Build history of the part. All positions in model axes, mm. A direction names the side the tool comes from. Give positions to 0.01 mm unless a question says otherwise; leave off trailing zeros. Order: outer loops, then holes, each group sorted by start corner. A loop starts at its lowest first (then second) coordinate and runs counter-clockwise, first axis right, second up. Notation, with made-up numbers: M -33,-30.5 L -15,-30.5 A28 ccw -15,-0.5 Z; hole C -22,57 d2. An arc over 180 degrees is marked long. One line per item, written item: value.
from build123d import *

# Parameters (mm, degrees)
BOSS_EXTRUDE1_DEPTH = 340


with BuildPart() as part:
    # Sketch1 → Boss-Extrude1 (new body)
    with BuildSketch(Plane(origin=(0, 0, 0), x_dir=(1, 0, 0), z_dir=(0, 1, 0))):
        with BuildLine():
            Line((-27.499872145, 29.213153277), (-67.499872145, 29.213153277))
            Line((-67.499872145, 29.213153277), (-67.499872145, -10.786846723))
            Line((-67.499872145, -10.786846723), (-66.499872145, -10.786846723))
            ThreePointArc((-66.499872145, -10.786846723), (-64.378551801, -9.908167067), (-63.499872145, -7.786846723))
            Line((-63.499872145, -7.786846723), (-63.499872145, 22.213153277))
            ThreePointArc((-63.499872145, 22.213153277), (-62.621192489, 24.334473621), (-60.499872145, 25.213153277))
            Line((-60.499872145, 25.213153277), (-30.499872145, 25.213153277))
            ThreePointArc((-30.499872145, 25.213153277), (-28.378551801, 26.091832933), (-27.499872145, 28.213153277))
            Line((-27.499872145, 28.213153277), (-27.499872145, 29.213153277))
        make_face()
    extrude(amount=BOSS_EXTRUDE1_DEPTH)


solid = part.part
1) Saw through at C-C, the plane z = -19. Write the cut outline in (x, y), then the cut area to 3 significant figures.
Check values:
outline: M -67.5,0 L -63.5,0 L -63.5,340 L -67.5,340 Z
area: 1,360 mm^2
2) Saw through at B-B, the plane x = -43. Write the cut outline in (y, z), then the cut area to 3 significant figures.
Check values:
outline: M 0,-29.21 L 340,-29.21 L 340,-25.21 L 0,-25.21 Z
area: 1,360 mm^2
3) Saw through at A-A, the plane y = 185. Write the cut outline in (x, z).
Check values:
outline: M -67.5,-29.21 L -27.5,-29.21 L -27.5,-28.21 A3 ccw -30.5,-25.21 L -60.5,-25.21 A3 cw -63.5,-22.21 L -63.5,7.79 A3 ccw -66.5,10.79 L -67.5,10.79 Z
4) Pin check, flat tips, straight feed: pin 1 (15 mm diameter, centred on x = -49.5, y = 169.5, fed in from +Z); pin 2 (10 mm diameter, centred on y = 196.5, z = 2, fed in from +X); pin 3 (24 mm diameter, centred on y = 224, z = -11.5, fed in from +X). Stop position of each tip, or through.
Check values:
pin 1: z = -25.21
pin 2: x = -63.5
pin 3: x = -63.21
5) Tool access for faces 1 (the face through (-67.5, 168, -9)), 2 (the face through (-63.5, 168, -7)): list every direction of +Z, -Z, +X, -X, +Y, -Y with a clear straight run to the whole face (end or side of a thin tool).
Check values:
face 1: +Z, -Z, -X, +Y, -Y
face 2: +Z, +X, +Y, -Y
6) Drill centre lines: probe 1 along Z at (x, y) = (-59, 218); probe 2 along X at (y, z) = (170.5, -5.5); probe 3 along Z at (x, y) = (-63, 142). Where is each one in solid material? Low to high. Write a range as from..to.
Check values:
probe 1: -29.21..-25.21
probe 2: -67.5..-63.5
probe 3: -29.21..-23.87
